Can you work these out from the model? Positions are in its coordinate system, mm. A direction names the side the tool comes from. Coordinates: 2 decimals unless noted, no trailing zeros. Order: outer loops, then holes, each group sorted by start corner. A loop starts at its lowest first (then second) coordinate and runs counter-clockwise, first axis right, second up. Notation, with made-up numbers: (75, 40.5) -> (91, 40.5) arc R32 ccw to (91, 72.5) -> close; hole circle Ø1 at (17, -0.75). An arc over 180 degrees is marked (long way). Answer in a Markdown table with one row per item. Add a question column.
1. Will these pins go through, and if not, where does the flat tip stop? pin 1 (1.5 mm diameter, centred on x = 1, y = 1, fed in from -Z); pin 2 (1 mm diameter, centred on x = 5, y = 0.5, fed in from -Z).
2. On a 3-axis mill with a long thin cutter (end or side, diameter ignored), from which of +Z, -Z, +X, -X, +Y, -Y can I reach the whole of each face in a straight line? I mean faces 1 (the face through (10, 0, 0)), 2 (the face through (6, 1, 0)), 3 (the face through (0.381, -0.137, -0.425)). Say none if no direction works.
3. We'd pull the mould along Z, two halves only. Please class faces 4 (the face through (0, 0.5, -0.5)), 5 (the face through (1.838, -0.26, 0.826)), 6 (the face through (0.381, 0.137, 0.425)): pulls with the +Z half, pulls with the -Z half, needs draft (parallel to the pull), parting line crosses it, or undercut.
4. If I drill on line 1 along Z through (x, y) = (6.5, -0.5); line 2 along Y through (x, z) = (8.5, -0.05); line 3 along Z through (x, y) = (0.5, -0.5), over which ranges is the centre line in solid material (lowest first)? Write a range as [from, to].
5. Imagine slicing it at B-B on x = 7.5. Write out the boundary of the cut face in (y, z), plus the area to 3 significant figures.
6. Imagine slicing it at A-A on x = 1. Write out the boundary of the cut face in (y, z), plus the area to 3 significant figures.
from build123d import *

# Parameters (mm, degrees)
PATTERN_CIRCULAR_1_COUNT = 2
PATTERN_CIRCULAR_1_ANGLE = 90


with BuildPart() as part:
    # 草图1 → Revolve 766 (revolve)
    with BuildSketch(Plane.XY, mode=Mode.PRIVATE) as revolve_766_sk:
        with BuildLine():
            Line((0, 0), (0, 2.2))
            Line((0, 2.2), (0.012446609, 2.2))
            Line((0.012446609, 2.2), (1.2, 1.012446609))
            ThreePointArc((1.2, 1.012446609), (1.362211674, 0.904060234), (1.553553391, 0.866))
            Line((1.553553391, 0.866), (2.114351801, 0.866))
            Line((2.114351801, 0.866), (2.346446609, 1))
            Line((2.346446609, 1), (10, 1))
            Line((10, 1), (10, 0))
            Line((10, 0), (0, 0))
        make_face()
    revolve(revolve_766_sk.sketch.rotate(Axis((0, 0, 0), (1, 0, 0)), 90), axis=Axis((0, 0, 0), (1, 0, 0)))

    # 草图2 → 切除-旋转1 (revolve, cut)
    with BuildSketch(Plane.XY, mode=Mode.PRIVATE) as cut_revolve_1_sk:
        Polygon((9.802166402, 1), (10.202166402, 1), (10, 0.6536), align=None)
    revolve(cut_revolve_1_sk.sketch.rotate(Axis((0, 0, 0), (-1, 0, 0)), 270), axis=Axis((0, 0, 0), (-1, 0, 0)), mode=Mode.SUBTRACT)

    # 草图3 → 切除-放样1 section 0
    with BuildSketch(Plane.ZY, mode=Mode.PRIVATE) as loft_1_s0:
        with BuildLine():
            Line((-1.1, 0.2), (1.1, 0.2))
            Line((1.1, 0.2), (1.1, -0.2))
            Line((1.1, -0.2), (-1.1, -0.2))
            Line((-1.1, -0.2), (-1.1, 0.2))
        make_face()
    loft_1 = loft([loft_1_s0.sketch, Vertex(1.2, 0, 0)], mode=Mode.SUBTRACT)

    # 阵列(圆周)1: 切除-放样1 ×2 about axis
    pattern_circular_1_axis = Axis((0, 0, 0), (1, 0, 0))
    for i in range(1, PATTERN_CIRCULAR_1_COUNT):
        add(loft_1.rotate(pattern_circular_1_axis, i * PATTERN_CIRCULAR_1_ANGLE / (PATTERN_CIRCULAR_1_COUNT - 1)), mode=Mode.SUBTRACT)


solid = part.part
Answers follow:
| question | item | result |
|---|---|---|
| 1 | pin 1 | stops at z = -1.77 |
| 1 | pin 2 | stops at z = -1 |
| 2 | face 1 | +Z, -Z, +X, +Y, -Y |
| 2 | face 2 | +X |
| 2 | face 3 | -X |
| 3 | face 4 | needs draft |
| 3 | face 5 | parting line crosses it |
| 3 | face 6 | undercut |
| 4 | line 1 | z = [-0.87, 0.87] |
| 4 | line 2 | y = [-1, 1] |
| 4 | line 3 | z = [-1.64, -0.12], [0.12, 1.64] |
| 5 | outline | circle Ø2 at (0, 0) |
| 5 | area | 3.14 mm² |
| 6 | outline | circle Ø2.42 at (0, 0); hole (-0.18, -0.03) -> (-0.03, -0.03) -> (-0.03, -0.18) -> (0.03, -0.18) -> (0.03, -0.03) -> (0.18, -0.03) -> (0.18, 0.03) -> (0.03, 0.03) -> (0.03, 0.18) -> (-0.03, 0.18) -> (-0.03, 0.03) -> (-0.18, 0.03) -> close |
| 6 | area | 4.57 mm² |
